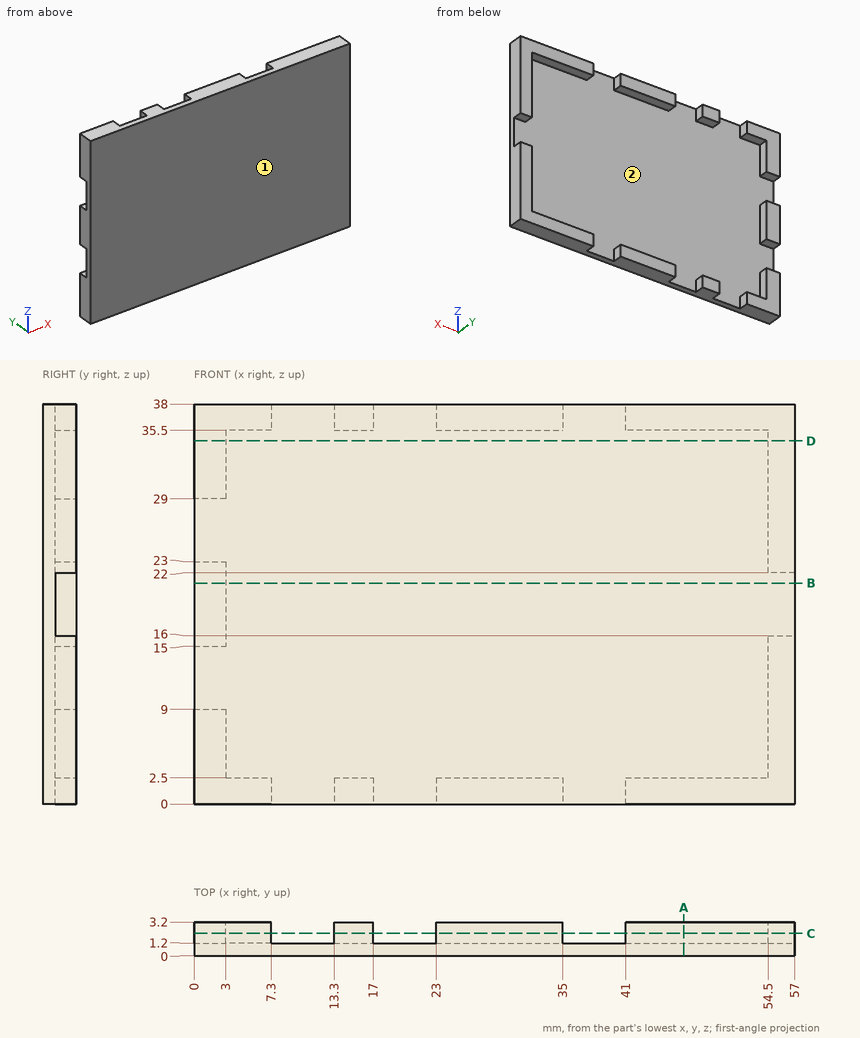
Geometry check sheet. Reference: drawing and pictorial views, mm from the part's lowest x, y, z. Coordinates: 2 decimals unless noted, no trailing zeros. Loops run counter-clockwise (first coordinate to the right, second up) from the corner with the lowest first, then second, coordinate; pieces in that order, holes last. Notation, with made-up numbers: (21.25, 19) - (72.25, 19) arc R24 cw to (72.25, 36) - close; hole circle Ø7 at (8, 84). An arc over 180 degrees is marked (long way). Return JSON: item names as keys, results as strings.
1. Go/stop test with flat-tipped pins: pin 1 (1.6 mm diameter, centred on y = 2.5, z = 37, fed in from -X); pin 2 (1 mm diameter, centred on x = 13, z = 7.5, fed in from +Y). Record where each tip stops, or that it passes through.
Established:
{"pin 1": "stops at x = 0", "pin 2": "stops at y = 1.2"}
2. Section check B-B, the plane z = 21. Record the boundary of the cut face in (x, y).
Established:
{"outline": "(0, 0) - (57, 0) - (57, 1.2) - (3, 1.2) - (3, 3.2) - (0, 3.2) - close"}
3. Section check A-A, the plane x = 46.5. Record the boundary of the cut face in (y, z), then the cut area to 3 significant figures.
Established:
{"outline": "(0, 0) - (3.2, 0) - (3.2, 2.5) - (1.2, 2.5) - (1.2, 35.5) - (3.2, 35.5) - (3.2, 38) - (0, 38) - close", "area": "55.6 mm2"}
4. Mould release check, pull along Z, two halves, no side actions. Record for the marked faces 1 and 2: +Z half, -Z half, draft (parallel to the pull), parting line (faces both ways), or undercut.
Established:
{"face 1": "draft", "face 2": "undercut"}
5. Section check D-D, the plane z = 34.5. Record the boundary of the cut face in (x, y), then the cut area to 3 significant figures.
Established:
{"outline": "(0, 0) - (57, 0) - (57, 3.2) - (54.5, 3.2) - (54.5, 1.2) - (3, 1.2) - (3, 3.2) - (0, 3.2) - close", "area": "79.4 mm2"}
6. Thickness scan on L1, parallel to Z at x = 16, y = 2.4; L2, parallel to X at y = 1.6, z = 22.5; L3, parallel to Y at x = 48, z = 7. Record the ranges inside material, lowest first.
Established:
{"L1": "z = 0 to 2.5, 35.5 to 38", "L2": "x = 0 to 3, 54.5 to 57", "L3": "y = 0 to 1.2"}
7. Section check C-C, the plane y = 2.15. Count the separate pieces of the cut face and the enclosed holes in it, then the cut area to 4 significant figures.
Established:
{"separate pieces": "9", "enclosed holes": "0", "area": "325.5 mm2"}
